Autodesk Inventor part; units mm, degrees
ref_plane "YZ Plane" through (0, 0, 0) normal (1, 0, 0) x (0, 1, 0)
ref_plane "XZ Plane" through (0, 0, 0) normal (0, 1, 0) x (-1, 0, 0)
ref_plane "XY Plane" through (0, 0, 0) normal (0, 0, 1) x (1, 0, 0)
sketch "Sketch1" plane through (0, 0, 0) normal (0, 0, 1) x (1, 0, 0)
  line L0 (0, -10) -> (25.4, -10)
  line L1 (25.4, 0) -> (0, 0)
  line L2 (0, 0) -> (0, -10)
  circle A0 centre (42.7, 70) radius 11.3
  arc A1 (51.5714, 84.8522) -> (49.2048, 53.9695) centre (42.7, 70) ccw
  arc A2 (25.4, -10) -> (51.5714, 84.8522) centre (25.4, 41.0367) ccw
  arc A3 (66.3907, 42.9781) -> (49.2048, 53.9695) centre (53.9047, 42.3867) ccw
  arc A4 (25.4, 0) -> (66.3907, 42.9781) centre (25.4, 41.0367) ccw
  point P0 (0, 0)
  point P1 (12.7, -10)
  point P2 (12.7, 0)
extrude "Extrusion1" add sketch "Sketch1" along normal blind 20
chamfer "Chamfer2" distance 2 angle 45 2 edges at (31.4, 70, 20) (31.4, 70, 0)
properties part number "tablet_arm_joint"
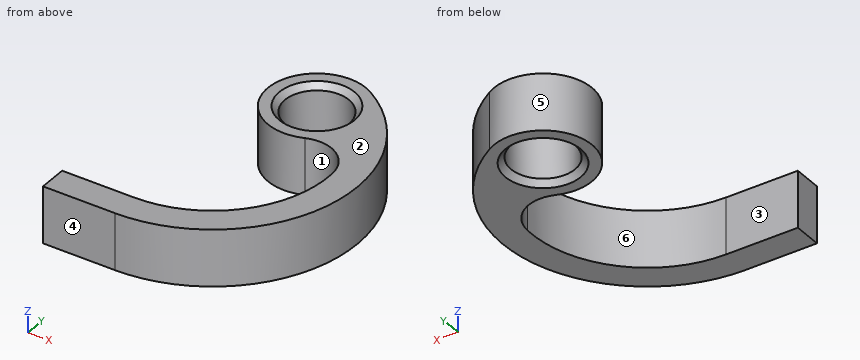
Verification items for the finished model (mm, model axes). Face numbers are marked on the shaded views. A direction names the side the tool comes from. Give positions to 0.01 mm unless a question says otherwise; leave off trailing zeros. Loops run counter-clockwise (first coordinate to the right, second up) from the corner with the lowest first, then second, coordinate; pieces in that order, holes last. Notation, with made-up numbers: M -7.75,65.5 L 6.25,65.5 A22 cw 6.25,77.5 Z; hole C -1,55 d1. An arc over 180 degrees is marked long. Return JSON: item names as keys, results as strings.
1) Section check A-A, the plane z = 12.75. Enter the section's corners in (x, y).
Findings:
{"outline": "M 0,-10 L 25.4,-10 A51.04 ccw 51.57,84.85 A17.3 ccw long 49.2,53.97 A12.5 cw 66.39,42.98 A41.04 cw 25.4,0 L 0,0 Z; hole C 42.7,70 d22.6"}
2) Section check C-C, the plane y = 70. Enter the section's corners in (x, z).
Findings:
{"outline": "M 25.4,0 L 29.4,0 L 31.4,2 L 31.4,18 L 29.4,20 L 25.4,20 Z; M 54,2 L 56,0 L 67.42,0 L 67.42,20 L 56,20 L 54,18 Z"}
3) Tool access check on the marked faces 1 and 2. Record the directions out of +Z, -Z, +X, -X, +Y, -Y that give a thin tool (end or side, any length) a straight path to the whole face; none if there is none.
Findings:
{"face 1": "+Z, -Z", "face 2": "+Z, +X, -X, +Y, -Y"}
4) Gauge pin test, flat ends, axial feed: P1, Ø4, axis at x = 59, z = 4.5, coming from the -Y side; P2, Ø8, axis at x = 9, z = 9, coming from the +Y side; P3, Ø13.5, axis at x = 42.7, y = 70, coming from the -Z side; P4, Ø2, axis at x = 43.5, z = 11, coming from the -Y side. Record the tip position at first contact, or that the pin passes through.
Findings:
{"P1": "stops at y = 0.96", "P2": "stops at y = 0", "P3": "passes through", "P4": "stops at y = -7.05"}
5) Section check B-B, the plane x = 42.7. Enter the section's corners in (y, z), and give its area (3 significant figures).
Findings:
{"outline": "M -6.98,0 L 3.82,0 L 3.82,20 L -6.98,20 Z; M 52.7,0 L 56.7,0 L 58.7,2 L 58.7,18 L 56.7,20 L 52.7,20 Z; M 81.3,2 L 83.3,0 L 87.3,0 L 87.3,20 L 83.3,20 L 81.3,18 Z", "area": "448 mm2"}
6) Section check D-D, the plane x = 23. Enter the section's corners in (y, z).
Findings:
{"outline": "M -10,0 L 0,0 L 0,20 L -10,20 Z"}
7) Mould release check, pull along Y, two halves, no side actions. Record for the marked faces 3, 4, 5 and 6: released by +Y, released by -Y, zero draft, split by the parting line, or undercut.
Findings:
{"face 3": "released by +Y", "face 4": "released by -Y", "face 5": "undercut", "face 6": "undercut"}
8) Material ranges on L1, parallel to Y at x = 42.7, z = 6.75; L2, parallel to Y at x = 43.5, z = 10.25; L3, parallel to X at y = 80, z = 5.5, recorded low to high. Write a range as [from, to].
Findings:
{"L1": "y = [-6.98, 3.82], [52.7, 58.7], [81.3, 87.3]", "L2": "y = [-6.68, 4.21], [52.72, 58.73], [81.27, 87.28]", "L3": "x = [28.58, 37.44], [47.96, 58.36]"}
